```python
from build123d import *

# Parameters (mm, degrees)
BOSS_EXTRUDE1_DEPTH   = 19.05
CUT_EXTRUDE1_DEPTH    = 219.215212878
CUT_EXTRUDE2_DEPTH    = 12.7
BOSS_EXTRUDE2_DEPTH   = 19.05
FILLET1_R             = 6.35
F_8_CLEARANCE_HOLE1_D = 4.3053


with BuildPart() as part:
    # Sketch1 → Boss-Extrude1 (new body)
    with BuildSketch(Plane(origin=(0, 0, 0), x_dir=(1, 0, 0), z_dir=(0, 1, 0))):
        with BuildLine():
            Line((-47.453228006, 53.404284402), (-98.253228006, 141.392465427))
            ThreePointArc((-98.253228006, 141.392465427), (-82.921975522, 181.453316928), (-41.566473575, 192.839342769))
            ThreePointArc((-41.566473575, 192.839342769), (36.836225704, 136.004392842), (45.380299153, 39.546144899))
            Line((45.380299153, 39.546144899), (27.944541838, -9.861512816))
            Line((27.944541838, -9.861512816), (0, 0))
            Line((0, 0), (-43.950457827, 15.509934128))
            ThreePointArc((-43.950457827, 15.509934128), (-41.550098289, 34.840876427), (-47.453228006, 53.404284402))
        make_face()
    extrude(amount=BOSS_EXTRUDE1_DEPTH)

    # Sketch5 → Cut-Extrude1 (cut, through all)
    with BuildSketch(Plane(origin=(0, 19.05, 0), x_dir=(1, 0, 0), z_dir=(0, 1, 0))):
        with BuildLine():
            Line((-29.23664893, 81.427581144), (15.574383155, 98.792652007))
            ThreePointArc((15.574383155, 98.792652007), (22.053436092, 98.460407789), (26.120098061, 93.405630482))
            ThreePointArc((26.120098061, 93.405630482), (31.67419382, 55.261505814), (28.616328902, 16.836622098))
            Line((28.616328902, 16.836622098), (22.559524164, 18.974043348))
            ThreePointArc((22.559524164, 18.974043348), (19.726825076, 6.545871538), (15.949337201, -5.628454892))
            Line((15.949337201, -5.628454892), (-31.95525319, 11.276876204))
            ThreePointArc((-31.95525319, 11.276876204), (-28.372538305, 23.563648828), (-26.173781301, 36.171824553))
            Line((-26.173781301, 36.171824553), (-32.322028113, 38.341515332))
            ThreePointArc((-32.322028113, 38.341515332), (-31.887912186, 55.427050363), (-34.131380562, 72.370214577))
            ThreePointArc((-34.131380562, 72.370214577), (-33.353370645, 77.801041885), (-29.23664893, 81.427581144))
        make_face()
    extrude(amount=-CUT_EXTRUDE1_DEPTH, mode=Mode.SUBTRACT)

    # Sketch6 → Cut-Extrude2 (cut)
    with BuildSketch(Plane(origin=(0, 19.05, 0), x_dir=(1, 0, 0), z_dir=(0, 1, 0))):
        with BuildLine():
            Line((-34.136031583, 72.371811773), (26.116293886, 93.401758977))
            add(Edge.make_bspline(
                [(26.116293886, 93.401758977), (24.324889601, 100.23803776), (22.130168151, 106.901258397), (16.96212823, 119.893613822), (13.988046064, 126.222420918), (9.776956475, 133.921680991), (8.910007749, 135.450921337), (7.126151123, 138.487965199), (6.207974968, 139.997768114), (3.386426272, 144.480432789), (1.42392697, 147.394611788), (-4.701484626, 155.920269738), (-9.100754748, 161.316287945), (-13.809441186, 166.430246232)],
                knots=[0, 0, 0, 0, 0.25, 0.25, 0.5, 0.5, 0.5625, 0.5625, 0.625, 0.625, 0.75, 0.75, 1, 1, 1, 1], degree=3))
            add(Edge.make_bspline(
                [(-26.604572492, 164.8773905), (-26.150591479, 165.703254328), (-25.515446259, 166.400295605), (-24.879031904, 167.098729697), (-24.095373437, 167.628794259), (-23.313760397, 168.1574753), (-22.428907317, 168.488425961), (-21.547481327, 168.818094831), (-20.612298709, 168.932538075), (-19.674896196, 169.047252981), (-18.735576663, 168.938540794), (-17.797334242, 168.829953267), (-16.909699728, 168.503685222), (-16.026331795, 168.178985445), (-15.242553256, 167.655985099), (-14.452846951, 167.129029268), (-13.809441186, 166.430246232)],
                knots=[0, 0, 0, 0.125, 0.125, 0.25, 0.25, 0.375, 0.375, 0.5, 0.5, 0.625, 0.625, 0.75, 0.75, 0.875, 0.875, 1, 1, 1], degree=2))
            Line((-26.604572492, 164.8773905), (-51.39264493, 119.783935416))
            add(Edge.make_bspline(
                [(-50.971516495, 111.453693883), (-51.597295758, 112.361285599), (-51.952278538, 113.405618938), (-52.307499269, 114.450652309), (-52.364051333, 115.554155451), (-52.420577964, 116.657162304), (-52.173441916, 117.734834771), (-51.926064332, 118.813560494), (-51.39264493, 119.783935416)],
                knots=[0, 0, 0, 0.25, 0.25, 0.5, 0.5, 0.75, 0.75, 1, 1, 1], degree=2))
            add(Edge.make_bspline(
                [(-50.971516495, 111.453693883), (-48.958817602, 108.534599247), (-47.092599274, 105.523689489), (-43.653878745, 99.317766492), (-42.08164257, 96.122586505), (-39.950407344, 91.187456603), (-39.27814351, 89.518531936), (-38.021441634, 86.160956199), (-37.435479748, 84.468826365), (-36.34793939, 81.058006993), (-35.846327383, 79.339328012), (-34.927561091, 75.875386956), (-34.510190541, 74.129079907), (-34.136031583, 72.371811773)],
                knots=[0, 0, 0, 0, 0.25, 0.25, 0.5, 0.5, 0.625, 0.625, 0.75, 0.75, 0.875, 0.875, 1, 1, 1, 1], degree=3))
        make_face()
    extrude(amount=-CUT_EXTRUDE2_DEPTH, mode=Mode.SUBTRACT)

    # Sketch7 → Boss-Extrude2 (add)
    with BuildSketch(Plane(origin=(0, 0, 0), x_dir=(1, 0, 0), z_dir=(0, 1, 0))):
        Polygon((-43.950457827, 15.509934128), (-52.403123375, -8.442361068), (-40.408086707, -12.675359716), (-31.95525319, 11.276876204), align=None)
    extrude(amount=BOSS_EXTRUDE2_DEPTH)

    # Fillet1
    fillet1_edges = [part.edges().sort_by_distance(p)[0] for p in [
        (-98.253228006, 9.525, -141.392465427),
        (27.944541838, 9.525, 9.861512816),
        (-52.403123375, 9.525, 8.442361068),
        (-40.408086707, 9.525, 12.675359716),
    ]]
    fillet(fillet1_edges, radius=FILLET1_R)

    # #8 Clearance Hole1 (through all)
    with Locations(Plane(origin=(0, 0, 0), x_dir=(-1, 0, 0), z_dir=(0, -1, 0))):
        with Locations((46.39038303, 115.861048868), (19.884364695, 162.99531268)):
            Hole(F_8_CLEARANCE_HOLE1_D / 2)


solid = part.part
```
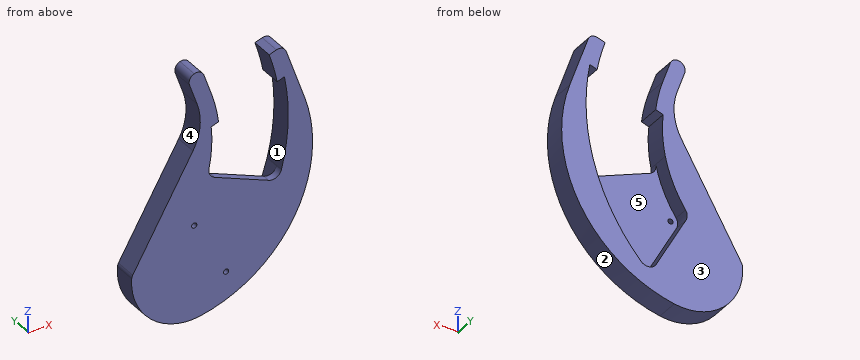
The model under review builds one solid part; all positions refer to its coordinate system, in mm. Face numbers are marked on the shaded views. A direction names the side the tool comes from. Give positions to 0.01 mm unless a question says otherwise; leave off trailing zeros. Write each loop counter-clockwise with the first axis right and the second up, starting at its lowest first coordinate (ties: lowest second). Pieces come first, ordered by that corner, then holes. Notation, with made-up numbers: M -3,77 L 23,77 A14 ccw 23,103 Z; hole C 85.25,61 d7. An arc over 180 degrees is marked long. Write item = value, one per line. Start each with the question number.
Q1. Mouldability with a two-part tool opening along Z and no side actions: class the marked faces 1, 2 and 3 as released by +Z, released by -Z, zero draft, split by the parting line, or undercut.
Q2. Clearance check with flat-ended pins moving along their axes: pin 1 (1.5 mm diameter, centred on y = 3.5, z = -151.5, fed in from +X); pin 2 (10 mm diameter, centred on y = 4.5, z = -111.5, fed in from -X); pin 3 (2 mm diameter, centred on x = -79, y = 8.5, fed in from -Z); pin 4 (2.5 mm diameter, centred on x = -19.88, z = -163, fed in from +Y). State where each tip first meets the part, or that it passes through.
Q3. We need section A-A (z = -27). State the section outline as (x, y) points.
Q4. We need section B-B (y = 2.25). Give the number of separate pieces and of enclosed holes in the cut face, plus the area to 3 significant figures.
Q5. For line 1 (Y direction, x = -28.5, z = -131); line 2 (X direction, y = 5.5, z = -58), list the stretches that pass through material, from the lowest coordinate up.
Q6. We need section D-D (z = -70). State the section outline as (x, y) points.
Q7. We need section C-C (x = -59.5). State the section outline as (y, z) points, plus the area to 3 significant figures.
Q8. Machinability: for the marked faces 4 and 5, which of the approach directions +Z, -Z, +X, -X, +Y, -Y give a long, thin tool a straight path to every point of the face, cutting with its end or side? Answer none if there is none.
Result set:
q1.face_1 = undercut
q1.face_2 = split by the parting line
q1.face_3 = zero draft
q2.pin_1 = 26.92
q2.pin_2 = -83.88
q2.pin_3 = -185.36
q2.pin_4 = through
q3.outline = M -41.5,0 L -27.63,0 L -27.63,19.05 L -41.5,19.05 Z; M 30.27,0 L 40.95,0 L 40.95,19.05 L 30.27,19.05 Z
q4.separate_pieces = 1
q4.enclosed_holes = 2
q4.area = 14,800 mm2
q5.line_1 = 0 to 6.35
q5.line_2 = -50.11 to -32.06, 31.56 to 50.24
q6.outline = M -57.03,0 L -33.65,0 L -33.65,19.05 L -57.03,19.05 Z; M 30.56,0 L 51.73,0 L 51.73,19.05 L 30.56,19.05 Z
q7.outline = M 0,-193.01 L 19.05,-193.01 L 19.05,-74.27 L 0,-74.27 Z
q7.area = 2,260 mm2
q8.face_4 = -X, +Y, -Y
q8.face_5 = +Y
